The listing builds one solid part. Answer for the finished solid, in the listing's coordinates (mm). Give positions to 0.01 mm unless a question says otherwise; leave off trailing zeros. Loops run counter-clockwise (first coordinate to the right, second up) from the corner with the lowest first, then second, coordinate; pieces in that order, holes last. Notation, with made-up numbers: (-22, -3.5) - (6, -3.5) arc R7 ccw to (6, 6.5) - close; hole circle Ø5 at (69, -12.5). An arc over 180 degrees is marked (long way). Answer as CSV lines item,"result". Start each with the question number.
1) A cutting plane is placed at B-B (y = -3.25). Determine the outline of the cut face in (x, z), and give its area (3 significant figures).
2) Flat-ended cylindrical pins translate along their axes: pin 1 (1.5 mm diameter, centred on y = 1.5, z = -2.5, fed in from +X); pin 2 (1.8 mm diameter, centred on x = 0.5, z = 1, fed in from -Y); pin 3 (5 mm diameter, centred on x = -1, z = 5, fed in from +Y). Find the tip coordinate at first contact, or state that the pin passes through.
3) A cutting plane is placed at C-C (x = 0). Determine the outline of the cut face in (y, z), and give its area (3 significant figures).
4) Find the intervals of material crossed by line 1 along X through (y, z) = (-4.25, 0); line 2 along Z through (x, y) = (0.5, -3.75); line 3 along X through (y, z) = (-4.75, -1.5), in increasing order.
5) A cutting plane is placed at A-A (z = 0). Determine the outline of the cut face in (x, y), and give its area (3 significant figures).
6) For a pull along Z with two mould halves and no side action, classify faces 1 (the face through (0.9, -4.93, -2.86)), 2 (the face through (-3.86, 0.25, -5.04)), 3 (the face through (0, 0, 0)), 4 (the face through (3, -10, 1)) as pulls with the +Z half, pulls with the -Z half, needs draft (parallel to the pull), parting line crosses it, or undercut.
7) A cutting plane is placed at D-D (x = 4.25). Determine the outline of the cut face in (y, z).
```python
from build123d import *

# Parameters (mm, degrees)
SKETCH1_R           = 6.35
BOSS_EXTRUDE1_DEPTH = 0.5
DOME1_FACE_RADIUS   = 6.35
DOME1_HEIGHT        = 6.35
SKETCH2_R           = 4.45
SKETCH2_R_2         = 3
BOSS_EXTRUDE2_DEPTH = 10


with BuildPart() as part:
    # Sketch1 → Boss-Extrude1 (new body)
    with BuildSketch(Plane(origin=(0, 0, 0), x_dir=(1, 0, 0), z_dir=(0, 1, 0))):
        with Locations(Location((0, 0, 0), (0, 0, 270))):
            Circle(SKETCH1_R)
    extrude(amount=BOSS_EXTRUDE1_DEPTH)

    # Dome1: a dome of height H over a round flat face of radius A is a cap of a sphere of radius (A * A + H * H) / (2 * H)
    dome1_r = (DOME1_FACE_RADIUS * DOME1_FACE_RADIUS + DOME1_HEIGHT * DOME1_HEIGHT) / (2 * DOME1_HEIGHT)
    dome1_base = Plane((0, 0.5, 0), z_dir=(0, 1, 0))
    with Locations(dome1_base.offset(DOME1_HEIGHT - dome1_r)):
        dome1_ball = Sphere(dome1_r, mode=Mode.PRIVATE)
    add(split(dome1_ball, bisect_by=dome1_base, keep=Keep.TOP, mode=Mode.PRIVATE))

    # Sketch2 → Boss-Extrude2 (add)
    with BuildSketch(Plane.XZ):
        with Locations(Location((0, 0, 0), (0, 0, 90))):
            Circle(SKETCH2_R)
        with Locations(Location((0, 0, 0), (0, 0, 270))):
            Circle(SKETCH2_R_2, mode=Mode.SUBTRACT)
    extrude(amount=BOSS_EXTRUDE2_DEPTH)


solid = part.part
```
Ans:
1,outline,"circle Ø8.9 at (0, 0); hole circle Ø6 at (0, 0)"
1,area,"33.9 mm2"
2,pin 1,"x = 6.05"
2,pin 2,"y = 0"
2,pin 3,"y = 6.29"
3,outline,"(-10, -4.45) - (0, -4.45) - (0, -6.35) - (0.5, -6.35) arc R6.35 ccw to (0.5, 6.35) - (0, 6.35) - (0, 4.45) - (-10, 4.45) - (-10, 3) - (0, 3) - (0, -3) - (-10, -3) - close"
3,area,"98.7 mm2"
4,line 1,"-4.45 to -3, 3 to 4.45"
4,line 2,"-4.42 to -2.96, 2.96 to 4.42"
4,line 3,"-4.19 to -2.6, 2.6 to 4.19"
5,outline,"(-6.35, 0) - (-4.45, 0) - (-4.45, -10) - (-3, -10) - (-3, 0) - (3, 0) - (3, -10) - (4.45, -10) - (4.45, 0) - (6.35, 0) - (6.35, 0.5) arc R6.35 ccw to (-6.35, 0.5) - close"
5,area,"98.7 mm2"
6,face 1,"undercut"
6,face 2,"parting line crosses it"
6,face 3,"undercut"
6,face 4,"needs draft"
7,outline,"(-10, -1.32) - (0, -1.32) - (0, -4.72) - (0.5, -4.72) arc R4.72 ccw to (0.5, 4.72) - (0, 4.72) - (0, 1.32) - (-10, 1.32) - close"
